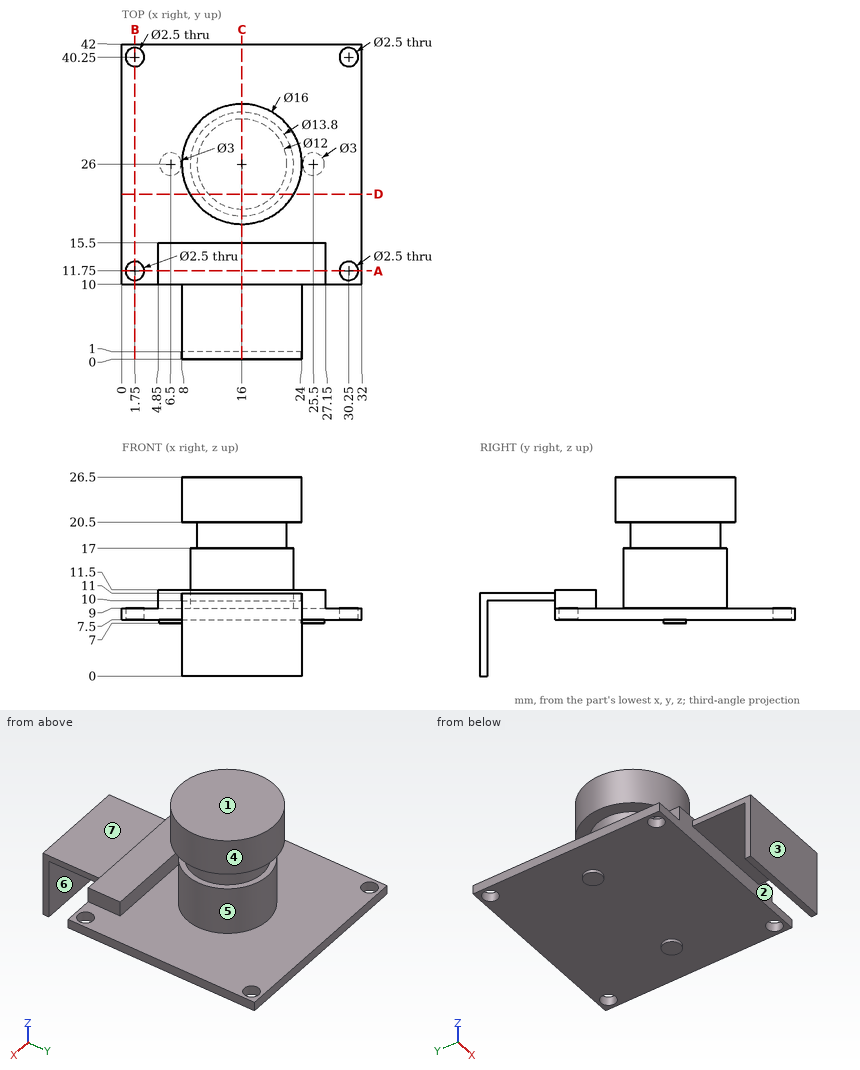
Check sheet for the drawn part. Datum: minimum x, y, z corner. Units: mm. A direction names the side the tool comes from. Coordinates: 2 decimals unless noted, no trailing zeros. Write each loop counter-clockwise with the first axis right and the second up, starting at its lowest first coordinate (ties: lowest second). Pieces come first, ordered by that corner, then holes. Notation, with made-up numbers: (-3.5, 77) - (42.5, 77) arc R31 ccw to (42.5, 115) - close; hole circle Ø6 at (-29, -16). An arc over 180 degrees is marked (long way). Answer as a JSON object with one key per item and string values.
(1) Cross-section at C-C on x = 16. Record the cut outline in (y, z), plus the area to 3 significant figures.
Report:
{"outline": "(0, 0) - (1, 0) - (1, 10) - (10, 10) - (10, 7.5) - (42, 7.5) - (42, 9) - (32.9, 9) - (32.9, 17) - (32, 17) - (32, 20.5) - (34, 20.5) - (34, 26.5) - (18, 26.5) - (18, 20.5) - (20, 20.5) - (20, 17) - (19.1, 17) - (19.1, 9) - (15.5, 9) - (15.5, 11.5) - (10, 11.5) - (10, 11) - (0, 11) - close", "area": "330 mm^2"}
(2) Thickness scan on line 1 along Y through (x, z) = (1.75, 8.4); line 2 along X through (y, z) = (40.25, 8.2); line 3 along Y through (x, z) = (23.5, 9.75). Record the ranges inside material, lowest first.
Report:
{"line 1": "10 to 10.5, 13 to 39, 41.5 to 42", "line 2": "0 to 0.5, 3 to 29, 31.5 to 32", "line 3": "0 to 1, 10 to 15.5"}
(3) Gauge pin test, flat ends, axial feed: pin 1 Ø2.5 at (x, y) = (25, 26.5) entering from -Z; pin 2 Ø8 at (x, y) = (13, 5.5) entering from +Z; pin 3 Ø4 at (x, y) = (30.25, 11.75) entering from +Z; pin 4 Ø8 at (x, z) = (14.5, 6.5) entering from +Y. Record the tip position at first contact, or that the pin passes through.
Report:
{"pin 1": "z = 7", "pin 2": "z = 11", "pin 3": "z = 9", "pin 4": "y = 42"}
(4) Mould release check, pull along Y, two halves, no side actions. Record for the marked faces 1, 2 and 3: pulls with the +Y half, pulls with the -Y half, needs draft (parallel to the pull), parting line crosses it, or undercut.
Report:
{"face 1": "needs draft", "face 2": "undercut", "face 3": "pulls with the -Y half"}
(5) Cross-section at B-B on x = 1.75. Record the cut outline in (y, z), plus the area to 3 significant figures.
Report:
{"outline": "(10, 7.5) - (10.5, 7.5) - (10.5, 9) - (10, 9) - close; (13, 7.5) - (39, 7.5) - (39, 9) - (13, 9) - close; (41.5, 7.5) - (42, 7.5) - (42, 9) - (41.5, 9) - close", "area": "40.5 mm^2"}
(6) Cross-section at D-D on y = 22. Record the cut outline in (x, z), plus the area to 3 significant figures.
Report:
{"outline": "(0, 7.5) - (32, 7.5) - (32, 9) - (21.62, 9) - (21.62, 17) - (20.47, 17) - (20.47, 20.5) - (22.93, 20.5) - (22.93, 26.5) - (9.07, 26.5) - (9.07, 20.5) - (11.53, 20.5) - (11.53, 17) - (10.38, 17) - (10.38, 9) - (0, 9) - close", "area": "252 mm^2"}
(7) Cross-section at A-A on y = 11.75. Record the cut outline in (x, z).
Report:
{"outline": "(0, 7.5) - (0.5, 7.5) - (0.5, 9) - (0, 9) - close; (3, 7.5) - (29, 7.5) - (29, 9) - (27.15, 9) - (27.15, 11.5) - (4.85, 11.5) - (4.85, 9) - (3, 9) - close; (31.5, 7.5) - (32, 7.5) - (32, 9) - (31.5, 9) - close"}
(8) Tool access check on the marked faces 4, 5, 6 and 7. Record the directions out of +Z, -Z, +X, -X, +Y, -Y that give a thin tool (end or side, any length) a straight path to the whole face; none if there is none.
Report:
{"face 4": "+Z", "face 5": "none", "face 6": "-Z, +X, -X", "face 7": "+Z, +X, -X, -Y"}
